Geometry check sheet. Reference: the model listing, model coordinates, mm. Face numbers are marked on the shaded views. A direction names the side the tool comes from. Round coordinates to 2 decimals unless told otherwise and drop trailing zeros. Write each loop counter-clockwise with the first axis right and the second up, starting at its lowest first coordinate (ties: lowest second). Pieces come first, ordered by that corner, then holes. Notation, with made-up numbers: (83, -33) -> (137, -33) arc R22 cw to (137, 6) -> close; hole circle Ø11 at (-19.5, 71.25). An arc over 180 degrees is marked (long way). Use a Markdown table: item, result.
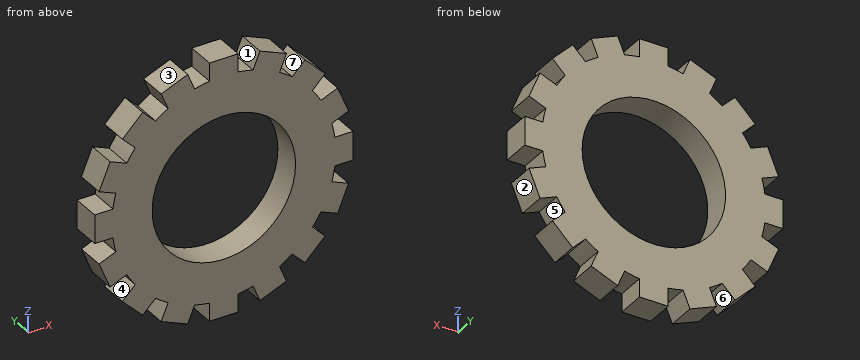
Autodesk Fusion 360 part; units mm, degrees
sketch "Sketch1" plane through (0, 0, 0) normal (0, 1, 0) x (1, 0, 0)
  circle A0 centre (0, 0) radius 25
  circle A1 centre (0, 0) radius 39
  line L0 (5, 45) -> (-5, 45)
  line L1 (-5, -45) -> (5, -45)
  line L2 (-5, 45) -> (-5, 38.6782)
  line L3 (-5, -38.6782) -> (-5, -45)
  line L4 (-5, 45) -> (-4.9694, 44.7248) construction
  line L5 (4.9694, -44.7248) -> (5, -45) construction
  line L6 (5, 45) -> (4.9694, 44.7248) construction
  line L7 (-4.9694, -44.7248) -> (-5, -45) construction
  line L8 (5, -45) -> (5, -38.6782)
  line L9 (5, 38.6782) -> (5, 45)
  line L10 (-10.1821, 37.6474) -> (-12.6014, 43.488)
  line L11 (-12.6014, 43.488) -> (-21.8402, 39.6612)
  line L12 (-21.8402, 39.6612) -> (-19.4209, 33.8205)
  line L13 (21.8402, -39.6612) -> (19.4209, -33.8205)
  line L14 (12.6014, -43.488) -> (21.8402, -39.6612)
  line L15 (10.1821, -37.6474) -> (12.6014, -43.488)
  line L16 (-23.8141, 30.8851) -> (-28.2843, 35.3553)
  line L17 (-28.2843, 35.3553) -> (-35.3553, 28.2843)
  line L18 (-35.3553, 28.2843) -> (-30.8851, 23.8141)
  line L19 (35.3553, -28.2843) -> (30.8851, -23.8141)
  line L20 (28.2843, -35.3553) -> (35.3553, -28.2843)
  line L21 (23.8141, -30.8851) -> (28.2843, -35.3553)
  line L22 (-33.8205, 19.4209) -> (-39.6612, 21.8402)
  line L23 (-39.6612, 21.8402) -> (-43.488, 12.6014)
  line L24 (-43.488, 12.6014) -> (-37.6474, 10.1821)
  line L25 (43.488, -12.6014) -> (37.6474, -10.1821)
  line L26 (39.6612, -21.8402) -> (43.488, -12.6014)
  line L27 (33.8205, -19.4209) -> (39.6612, -21.8402)
  line L28 (-38.6782, 5) -> (-45, 5)
  line L29 (-45, 5) -> (-45, -5)
  line L30 (-45, -5) -> (-38.6782, -5)
  line L31 (45, 5) -> (38.6782, 5)
  line L32 (45, -5) -> (45, 5)
  line L33 (38.6782, -5) -> (45, -5)
  line L34 (-37.6474, -10.1821) -> (-43.488, -12.6014)
  line L35 (-43.488, -12.6014) -> (-39.6612, -21.8402)
  line L36 (-39.6612, -21.8402) -> (-33.8205, -19.4209)
  line L37 (39.6612, 21.8402) -> (33.8205, 19.4209)
  line L38 (43.488, 12.6014) -> (39.6612, 21.8402)
  line L39 (37.6474, 10.1821) -> (43.488, 12.6014)
  line L40 (-30.8851, -23.8141) -> (-35.3553, -28.2843)
  line L41 (-35.3553, -28.2843) -> (-28.2843, -35.3553)
  line L42 (-28.2843, -35.3553) -> (-23.8141, -30.8851)
  line L43 (28.2843, 35.3553) -> (23.8141, 30.8851)
  line L44 (35.3553, 28.2843) -> (28.2843, 35.3553)
  line L45 (30.8851, 23.8141) -> (35.3553, 28.2843)
  line L46 (-19.4209, -33.8205) -> (-21.8402, -39.6612)
  line L47 (-21.8402, -39.6612) -> (-12.6014, -43.488)
  line L48 (-12.6014, -43.488) -> (-10.1821, -37.6474)
  line L49 (12.6014, 43.488) -> (10.1821, 37.6474)
  line L50 (21.8402, 39.6612) -> (12.6014, 43.488)
  line L51 (19.4209, 33.8205) -> (21.8402, 39.6612)
  line L52 (-5, -38.6782) -> (-5, -45)
  line L53 (-5, -45) -> (5, -45)
  line L54 (5, -45) -> (5, -38.6782)
  line L55 (-5, 45) -> (-5, 38.6782)
  line L56 (5, 45) -> (-5, 45)
  line L57 (5, 38.6782) -> (5, 45)
  line L58 (10.1821, -37.6474) -> (12.6014, -43.488)
  line L59 (12.6014, -43.488) -> (21.8402, -39.6612)
  line L60 (21.8402, -39.6612) -> (19.4209, -33.8205)
  line L61 (-21.8402, 39.6612) -> (-19.4209, 33.8205)
  line L62 (-12.6014, 43.488) -> (-21.8402, 39.6612)
  line L63 (-10.1821, 37.6474) -> (-12.6014, 43.488)
  line L64 (23.8141, -30.8851) -> (28.2843, -35.3553)
  line L65 (28.2843, -35.3553) -> (35.3553, -28.2843)
  line L66 (35.3553, -28.2843) -> (30.8851, -23.8141)
  line L67 (-35.3553, 28.2843) -> (-30.8851, 23.8141)
  line L68 (-28.2843, 35.3553) -> (-35.3553, 28.2843)
  line L69 (-23.8141, 30.8851) -> (-28.2843, 35.3553)
  line L70 (33.8205, -19.4209) -> (39.6612, -21.8402)
  line L71 (39.6612, -21.8402) -> (43.488, -12.6014)
  line L72 (43.488, -12.6014) -> (37.6474, -10.1821)
  line L73 (-43.488, 12.6014) -> (-37.6474, 10.1821)
  line L74 (-39.6612, 21.8402) -> (-43.488, 12.6014)
  line L75 (-33.8205, 19.4209) -> (-39.6612, 21.8402)
  line L76 (38.6782, -5) -> (45, -5)
  line L77 (45, -5) -> (45, 5)
  line L78 (45, 5) -> (38.6782, 5)
  line L79 (-45, -5) -> (-38.6782, -5)
  line L80 (-45, 5) -> (-45, -5)
  line L81 (-38.6782, 5) -> (-45, 5)
  line L82 (37.6474, 10.1821) -> (43.488, 12.6014)
  line L83 (43.488, 12.6014) -> (39.6612, 21.8402)
  line L84 (39.6612, 21.8402) -> (33.8205, 19.4209)
  line L85 (-39.6612, -21.8402) -> (-33.8205, -19.4209)
  line L86 (-43.488, -12.6014) -> (-39.6612, -21.8402)
  line L87 (-37.6474, -10.1821) -> (-43.488, -12.6014)
  line L88 (30.8851, 23.8141) -> (35.3553, 28.2843)
  line L89 (35.3553, 28.2843) -> (28.2843, 35.3553)
  line L90 (28.2843, 35.3553) -> (23.8141, 30.8851)
  line L91 (-28.2843, -35.3553) -> (-23.8141, -30.8851)
  line L92 (-35.3553, -28.2843) -> (-28.2843, -35.3553)
  line L93 (-30.8851, -23.8141) -> (-35.3553, -28.2843)
  line L94 (19.4209, 33.8205) -> (21.8402, 39.6612)
  line L95 (21.8402, 39.6612) -> (12.6014, 43.488)
  line L96 (12.6014, 43.488) -> (10.1821, 37.6474)
  line L97 (-12.6014, -43.488) -> (-10.1821, -37.6474)
  line L98 (-21.8402, -39.6612) -> (-12.6014, -43.488)
  line L99 (-19.4209, -33.8205) -> (-21.8402, -39.6612)
  dimension "d1" = 50
  dimension "d3" = 78
  dimension "d4" = 10
  dimension "d5" = 90
  dimension "d7" = 360
extrude "Extrude1" add sketch "Sketch1" along normal blind 10
(1) Release check for a two-part mould opening along X. For the marked faces 1, 2 and 3 record: +X half, -X half, draft (parallel to the pull), parting line (faces both ways), or undercut.
A:
| item | result |
|---|---|
| face 1 | undercut |
| face 2 | +X half |
| face 3 | -X half |
(2) Access from +Z, -Z, +X, -X, +Y, -Y to the whole of each face (thin tool, end or side, straight path). Record for the marked faces 4, 5, 6 and 7.
A:
| item | result |
|---|---|
| face 4 | -X, +Y, -Y |
| face 5 | +Y, -Y |
| face 6 | -Z, +Y, -Y |
| face 7 | +Z, +Y, -Y |
(3) Thickness scan on line 1 (X direction, y = 4.25, z = 0); line 2 (Z direction, x = 34.5, y = 3.5); line 3 (Z direction, x = 32, y = 7). Record the ranges inside material, lowest first.
A:
| item | result |
|---|---|
| line 1 | x = -45 to -25, 25 to 45 |
| line 2 | z = -29.14 to -27.43, -19.7 to 19.7, 27.43 to 29.14 |
| line 3 | z = -31.64 to -24.93, -22.29 to 22.29, 24.93 to 31.64 |
(4) Section check A-A on x = 0. Record the cut outline in (y, z).
A:
| item | result |
|---|---|
| outline | (0, -45) -> (10, -45) -> (10, -25) -> (0, -25) -> close; (0, 25) -> (10, 25) -> (10, 45) -> (0, 45) -> close |
(5) Gauge pin test, flat ends, axial feed: pin 1 Ø3 at (x, y) = (40.5, 3.5) entering from +Z; pin 2 Ø1.9 at (x, y) = (-41.5, 5) entering from +Z; pin 3 Ø1 at (x, y) = (7, 8) entering from -Z. Record the tip position at first contact, or that the pin passes through.
A:
| item | result |
|---|---|
| pin 1 | stops at z = 21.84 |
| pin 2 | stops at z = 19.69 |
| pin 3 | stops at z = -38.45 |
(6) Section check B-B on z = 0. Record the cut outline in (x, y), plus the area to 3 significant figures.
A:
| item | result |
|---|---|
| outline | (-45, 0) -> (-25, 0) -> (-25, 10) -> (-45, 10) -> close; (25, 0) -> (45, 0) -> (45, 10) -> (25, 10) -> close |
| area | 400 mm2 |
